```python
from build123d import *

# Parameters (mm, degrees)
F1_DEPTH = 25.4
F2_R     = 6.35
F3_DEPTH = 25.4
F5_DEPTH = 25.4
F7_DEPTH = 25.4


with BuildPart() as f1:
    # F0 (on Front) → F1 (new body)
    with BuildSketch(Plane.XZ):
        Polygon((0, 38.1), (0, 0), (69.85, 0), (69.85, 12.7), (25.4, 12.7), (25.4, 38.1), align=None)
    extrude(amount=F1_DEPTH)

    # F2 (on face) → F3 (cut)
    with BuildSketch(Plane.XZ.offset(25.4)):
        with Locations((12.7, 25.4)):
            Circle(F2_R)
    extrude(amount=-F3_DEPTH, mode=Mode.SUBTRACT)

    # F4 (on face) → F5 (cut)
    with BuildSketch(Plane.XZ.offset(25.4)):
        with BuildLine():
            ThreePointArc((0, 29.248118894), (3.3165566282, 34.7834433718), (8.851881106, 38.1))
            Line((8.851881106, 38.1), (0, 38.1))
            Line((0, 38.1), (0, 29.248118894))
        make_face()
        with BuildLine():
            ThreePointArc((16.548118894, 38.1), (22.0834433718, 34.7834433718), (25.4, 29.248118894))
            Line((25.4, 29.248118894), (25.4, 38.1))
            Line((25.4, 38.1), (16.548118894, 38.1))
        make_face()
    extrude(amount=-F5_DEPTH, mode=Mode.SUBTRACT)

    # F6 (on face) → F7 (cut)
    with BuildSketch(Plane.XY.offset(12.7)):
        with BuildLine():
            Line((38.209768584, -6.3509488222), (37.9895952922, -6.350959852))
            ThreePointArc((37.9895952922, -6.350959852), (31.7505322918, -12.7822181363), (38.1540299444, -19.0497701348))
            ThreePointArc((38.1540299444, -19.0497701348), (42.6091900684, -17.1709847826), (44.45, -12.7))
            ThreePointArc((44.45, -12.7), (42.6287708326, -8.2488501771), (38.209768584, -6.3509488222))
        make_face()
        with BuildLine():
            ThreePointArc((44.45, -12.7), (42.6091900684, -17.1709847826), (38.1540299444, -19.0497701348))
            Line((38.1540299444, -19.0497701348), (57.1499231602, -19.0499999995))
            ThreePointArc((57.1499231602, -19.0499999995), (50.8000000011, -12.700120635), (57.1496818903, -6.350000008))
            Line((57.1496818903, -6.350000008), (38.209768584, -6.3509488222))
            ThreePointArc((38.209768584, -6.3509488222), (42.6287708326, -8.2488501771), (44.45, -12.7))
        make_face()
        with BuildLine():
            ThreePointArc((57.1496818903, -6.350000008), (50.8000000011, -12.700120635), (57.1499231602, -19.0499999995))
            ThreePointArc((57.1499231602, -19.0499999995), (61.6401008935, -17.1901552274), (63.5, -12.7))
            ThreePointArc((63.5, -12.7), (61.6400155904, -8.2097594721), (57.1496818903, -6.350000008))
        make_face()
        with BuildLine():
            ThreePointArc((63.1413459778, 0), (67.4724972226, -12.7546630792), (62.8318339586, -25.4))
            Line((62.8318339586, -25.4), (69.85, -25.4))
            Line((69.85, -25.4), (69.85, 0))
            Line((69.85, 0), (63.1413459778, 0))
        make_face()
    extrude(amount=-F7_DEPTH, mode=Mode.SUBTRACT)


solid = f1.part
```
Check sheet for the modelled part. Datum: model origin and axes. Units: mm. A direction names the side the tool comes from. Round coordinates to 2 decimals unless told otherwise and drop trailing zeros. Order: outer loops, then holes, each group sorted by start corner. A loop starts at its lowest first (then second) coordinate and runs counter-clockwise, first axis right, second up. Notation, with made-up numbers: (41.25, 21) -> (48.25, 21) arc R13 ccw to (48.25, 30) -> close; hole circle Ø4 at (79, 82.5). An arc over 180 degrees is marked (long way). Use CSV: the item, a comma, the result in double quotes.
(1) Tool access check on faces 4 (the face through (47, -4, 12.7)), 5 (the face through (3.252, -12.878, 34.719)). Record the directions out of +Z, -Z, +X, -X, +Y, -Y that give a thin tool (end or side, any length) a straight path to the whole face; none if there is none.
Worked out:
face 4,"+Z, +X, +Y, -Y"
face 5,"+Z, -X, +Y, -Y"
(2) Cross-section at A-A (z = 9). Record the boundary of the cut face in (x, y), and give its area (3 significant figures).
Worked out:
outline,"(0, -25.4) -> (62.83, -25.4) arc R20.22 ccw to (63.14, 0) -> (0, 0) -> close; hole (37.99, -6.35) arc R6.35 ccw to (38.15, -19.05) -> (57.15, -19.05) arc R6.35 ccw to (57.15, -6.35) -> close"
area,"1,310 mm²"
(3) Cross-section at D-D (z = 27). Record the boundary of the cut face in (x, y).
Worked out:
outline,"(0, -25.4) -> (6.55, -25.4) -> (6.55, 0) -> (0, 0) -> close; (18.85, -25.4) -> (25.4, -25.4) -> (25.4, 0) -> (18.85, 0) -> close"
(4) Draft check along X on faces 1 (the face through (13, -13, 38.1)), 2 (the face through (25.4, -13, 21)), 3 (the face through (31.75, -12.64, 6.44)). Enter one of: pulls with the +X half, pulls with the -X half, needs draft (parallel to the pull), parting line crosses it, or undercut.
Worked out:
face 1,"needs draft"
face 2,"pulls with the +X half"
face 3,"undercut"
(5) Cross-section at C-C (x = 12.7). Record the boundary of the cut face in (y, z), and give its area (3 significant figures).
Worked out:
outline,"(-25.4, 0) -> (0, 0) -> (0, 19.05) -> (-25.4, 19.05) -> close; (-25.4, 31.75) -> (0, 31.75) -> (0, 38.1) -> (-25.4, 38.1) -> close"
area,"645 mm²"
(6) Depth check by flat-ended pin: pin 1 (12.5 mm diameter, centred on x = 46, y = -13, fed in from +Z); pin 2 (2 mm diameter, centred on x = 7, y = -7, fed in from +Z); pin 3 (13 mm diameter, centred on y = -7.5, z = 17, fed in from +X); pin 4 (7.5 mm diameter, centred on x = 12.7, z = 25.4, fed in from -Y). Enter the tip coordinate at first touch or a pass-through.
Worked out:
pin 1,"z = 12.7"
pin 2,"z = 37.81"
pin 3,"x = 67.47"
pin 4,"through"
(7) Material ranges on line 1 along Z through (x, y) = (12.7, -19.75); line 2 along Y through (x, z) = (49, 9); line 3 along Z through (x, y) = (48, -20.5), recorded low to high. Write a range as from..to.
Worked out:
line 1,"0..19.05, 31.75..38.1"
line 2,"-25.4..-19.05, -6.35..0"
line 3,"0..12.7"
(8) Cross-section at B-B (y = -12). Record the boundary of the cut face in (x, z), and give its area (3 significant figures).
Worked out:
outline,"(0, 0) -> (31.79, 0) -> (31.79, 12.7) -> (25.4, 12.7) -> (25.4, 29.25) arc R13.27 ccw to (16.55, 38.1) -> (8.85, 38.1) arc R13.27 ccw to (0, 29.25) -> close; (63.46, 0) -> (67.47, 0) -> (67.47, 12.7) -> (63.46, 12.7) -> close; hole circle Ø12.7 at (12.7, 25.4)"
area,"921 mm²"
